Here's how the part is built. I have some questions about the finished solid (model axes, mm). A direction names the side the tool comes from. Give positions to 0.01 mm unless a question says otherwise; leave off trailing zeros. Order: outer loops, then holes, each group sorted by start corner. A loop starts at its lowest first (then second) coordinate and runs counter-clockwise, first axis right, second up. Notation, with made-up numbers: (12.25, 11) - (47.25, 11) arc R13 cw to (47.25, 22) - close; hole circle Ø2 at (51, 11). An arc over 180 degrees is marked (long way). One line per question, with ' | ' between items.
from build123d import *

# Parameters (mm, degrees)
BOSS_EXTRUDE1_DEPTH = 1.5
CIRPATTERN1_COUNT   = 4
SKETCH5_R           = 2.25
CUT_EXTRUDE1_DEPTH  = 58.177142505
CUT_EXTRUDE2_DEPTH  = 3.2
CIRPATTERN2_COUNT   = 6


with BuildPart() as part:
    # Sketch2 → Revolve1 (revolve)
    with BuildSketch(Plane.XY, mode=Mode.PRIVATE) as revolve1_sk:
        Polygon((7, 25.525), (10, 25.525), (10, 15.525), (14.2, 15.525), (14.2, 6), (38, 6), (38, 0), (11.2, 0), (11.2, 7), (7, 7), align=None)
    revolve(revolve1_sk.sketch.rotate(Axis((0, 0, 0), (0, 1, 0)), 90), axis=Axis((0, 0, 0), (0, 1, 0)))

    # Sketch4 → Boss-Extrude1 (add, symmetric)
    with BuildSketch(Plane.XY):
        with BuildLine():
            Line((-7, 25.525), (-12.2, 25.525))
            ThreePointArc((-12.2, 25.525), (-13.672135955, 23.761067977), (-14.2, 21.525))
            Line((-14.2, 21.525), (-14.2, 15.525))
            Line((-14.2, 15.525), (-7, 15.525))
            Line((-7, 15.525), (-7, 25.525))
        make_face()
    boss_extrude1 = extrude(amount=BOSS_EXTRUDE1_DEPTH, both=True)

    # CirPattern1: Boss-Extrude1 ×4 about axis
    cirpattern1_axis = Axis((0, 0, 0), (0, 1, 0))
    for i in range(1, CIRPATTERN1_COUNT):
        add(boss_extrude1.rotate(cirpattern1_axis, i * 360 / CIRPATTERN1_COUNT))

    # Sketch5 → Cut-Extrude1 (cut, through all)
    with BuildSketch(Plane(origin=(0, 6, 0), x_dir=(1, 0, 0), z_dir=(0, 1, 0))):
        with Locations(Location((0, 25, 0), (0, 0, 270))):
            Circle(SKETCH5_R)
    cut_extrude1 = extrude(amount=-CUT_EXTRUDE1_DEPTH, mode=Mode.SUBTRACT)

    # Sketch6 → Cut-Extrude2 (cut)
    with BuildSketch(Plane.XZ):
        Polygon((4.156921938, -25), (2.078460969, -21.4), (-2.078460969, -21.4), (-4.156921938, -25), (-2.078460969, -28.6), (2.078460969, -28.6), align=None)
    cut_extrude2 = extrude(amount=-CUT_EXTRUDE2_DEPTH, mode=Mode.SUBTRACT)

    # CirPattern2: Cut-Extrude1, Cut-Extrude2 ×6 about axis
    cirpattern2_axis = Axis((0, 0, 0), (0, 1, 0))
    add([cut_extrude1.rotate(cirpattern2_axis, i * 360 / CIRPATTERN2_COUNT) for i in range(1, CIRPATTERN2_COUNT)], mode=Mode.SUBTRACT)
    add([cut_extrude2.rotate(cirpattern2_axis, i * 360 / CIRPATTERN2_COUNT) for i in range(1, CIRPATTERN2_COUNT)], mode=Mode.SUBTRACT)


solid = part.part
1) I'm going to push flat-ended pins straight in: P1, Ø3.5, axis at x = 0.5, y = 19, coming from the -Z side; P2, Ø3.5, axis at x = 21.5, y = 1.5, coming from the -Z side; P3, Ø6, axis at x = 21.65, z = 12.5, coming from the +Y side; P4, Ø3.5, axis at x = 21.65, z = -12.5, coming from the -Y side. Where does each tip first touch, or does it pass through?
Model answer:
P1: stops at z = -14.2 | P2: stops at z = -32.46 | P3: stops at y = 6 | P4: passes through
2) Thinking about a two-plate mould opening in X: for faces 5 (the face through (-20.13, 4.62, 10.84)), 6 (the face through (7.01, 20.45, 7.13)), 7 (the face through (-7.13, 20.45, 7.01)), which applies, +X half, -X half, draft (parallel to the pull), parting line (faces both ways), or undercut?
Model answer:
face 5: undercut | face 6: +X half | face 7: -X half
3) I want a section at A-A (z = -6). List the corners of the cut face in (x, y) for me (3 decimals).
Model answer:
outline: (-37.523, 0) - (-9.457, 0) - (-9.457, 7) - (-3.606, 7) - (-3.606, 25.525) - (-8, 25.525) - (-8, 15.525) - (-12.87, 15.525) - (-12.87, 6) - (-37.523, 6) - close; (3.606, 7) - (9.457, 7) - (9.457, 0) - (37.523, 0) - (37.523, 6) - (12.87, 6) - (12.87, 15.525) - (8, 15.525) - (8, 25.525) - (3.606, 25.525) - close
4) Please list where these lines run through material, in increasing order: L1, parallel to X at y = 4.05, z = -25; L2, parallel to X at y = 4.95, z = -12.5; L3, parallel to Z at x = 2.5, y = 3.
Model answer:
L1: x = -28.62 to -2.25, 2.25 to 28.62 | L2: x = -35.89 to -23.9, -19.4 to 19.4, 23.9 to 35.89 | L3: z = -37.92 to -27.87, -22.13 to -10.92, 10.92 to 22.13, 27.87 to 37.92
5) On a 3-axis mill with a long thin cutter (end or side, diameter ignored), from which of +Z, -Z, +X, -X, +Y, -Y can I reach the whole of each face in a straight line? I mean faces 1 (the face through (12, 21, -1.5)), 2 (the face through (0, 19, -14.2)), 3 (the face through (14.2, 19, 0)), 4 (the face through (-3, 2, 23)). Say none if no direction works.
Model answer:
face 1: -Z, +X, +Y | face 2: -Z, +X, -X, +Y | face 3: +Z, -Z, +X, +Y | face 4: -Y
